Input: part model. Units: mm. Frame: model coordinates. A direction names the side the tool comes from. Coordinates: 2 decimals unless noted, no trailing zeros. Write each loop counter-clockwise with the first axis right and the second up, starting at its lowest first coordinate (ties: lowest second). Pieces come first, ordered by that corner, then holes. Notation, with made-up numbers: (63, 56) - (93, 56) arc R13 ccw to (93, 80) - close; hole circle Ø9 at (16.5, 73). An arc over 180 degrees is marked (long way). Put each result on its own line as item: value. Start each with the question number.
1. Pin query (flat end, axial travel): pin 1 (2 mm diameter, centred on x = -62, z = -5.5, fed in from +Y); pin 2 (1.5 mm diameter, centred on x = -2, z = -2.5, fed in from +Y); pin 3 (3 mm diameter, centred on x = -38.5, z = 1.5, fed in from +Y). Return the tip coordinate at first contact, or that it passes through.
2. Cut plane D-D, the plane x = -17. Return loops of the section in (y, z).
3. Cut plane A-A, the plane x = -64.35. Return loops of the section in (y, z).
4. Line query: line 1 (Y direction, x = -64.35, z = -20.8); line 2 (Y direction, x = -26, z = -21); line 3 (Z direction, x = -65, y = 8). Output: solid intervals per line, ascending.
5. Access query for faces 4 (the flat face through (-36, 7, 0)), 5 (the flat face through (-44.668, 13.675, -22.535)), 6 (the flat face through (-67, 48, -21)). Directions: +Z, -Z, +X, -X, +Y, -Y. A direction counts if a zero-diameter tool reaches every point of the face in a straight line with its end or side. Return the directions, or none.
6. Cut plane B-B, the plane y = 52.5. Return loops of the section in (x, z), and give its area (3 significant figures).
7. Pull-direction query (Z, two-part tool) for faces 1 (the flat face through (-68.48, 25.97, -22.54)), 2 (the flat face through (-3, 10, -15)), 3 (the flat face through (-3, 13, 2)); classes: released by +Z, released by -Z, zero draft, split by the parting line, or undercut.
8. Cut plane C-C, the plane z = -1.5. Return loops of the section in (x, y).
from build123d import *

# Parameters (mm, degrees)
SKETCH2_W            = 70
SKETCH2_H            = 20
BOSS_EXTRUDE1_DEPTH  = 5
SKETCH3_W            = 70
SKETCH3_H            = 5
BOSS_EXTRUDE2_DEPTH  = 10
SKETCH4_W            = 5
SKETCH4_H            = 5
BOSS_EXTRUDE3_DEPTH  = 10
LOFT1_START          = -5
LOFT1_DEPTH          = 5
SKETCH7_W            = 3
SKETCH7_H            = 20
BOSS_EXTRUDE4_DEPTH  = 5
LOFT2_START          = -5
LOFT2_DEPTH          = 5
BOSS_EXTRUDE5_DEPTH  = 5
SKETCH12_W           = 46.347010245
SKETCH12_H           = 26.5
CUT_EXTRUDE1_DEPTH   = 14
BOSS_EXTRUDE6_DEPTH  = 5
BOSS_EXTRUDE7_DEPTH  = 5
SKETCH17_W           = 6.7
SKETCH17_H           = 6
BOSS_EXTRUDE8_DEPTH  = 5
SKETCH18_W           = 5.3
SKETCH18_H           = 6
BOSS_EXTRUDE9_DEPTH  = 5
SKETCH23_W           = 6.7
SKETCH23_H           = 2
SKETCH23_W_2         = 5.3
BOSS_EXTRUDE12_DEPTH = 10
SKETCH24_R           = 1.6
CUT_EXTRUDE4_DEPTH   = 10


# Read off the part's stored shape, not the designer's step: Loft1, Loft2
with BuildPart() as part:
    # Sketch2 → Boss-Extrude1 (new body)
    with BuildSketch(Plane(origin=(0, 0, 0), x_dir=(1, 0, 0), z_dir=(0, 1, 0))):
        with Locations((-35, 10)):
            Rectangle(SKETCH2_W, SKETCH2_H)
    extrude(amount=BOSS_EXTRUDE1_DEPTH)

    # Sketch3 → Boss-Extrude2 (add)
    with BuildSketch(Plane(origin=(0, 0, 0), x_dir=(1, 0, 0), z_dir=(0, 1, 0))):
        with Locations((-35, 22.5)):
            Rectangle(SKETCH3_W, SKETCH3_H)
        with Locations((-35, -2.5)):
            Rectangle(SKETCH3_W, SKETCH3_H)
    extrude(amount=BOSS_EXTRUDE2_DEPTH)

    # Sketch4 → Boss-Extrude3 (add)
    with BuildSketch(Plane(origin=(0, 5, 0), x_dir=(1, 0, 0), z_dir=(0, 1, 0))):
        with Locations((-2.5, 2.5)):
            Rectangle(SKETCH4_W, SKETCH4_H)
        with Locations((-2.5, 17.5)):
            Rectangle(SKETCH4_W, SKETCH4_H)
    extrude(amount=BOSS_EXTRUDE3_DEPTH)

    # Loft1 outline → Loft1 (add)
    with BuildSketch(Plane.YZ.offset(LOFT1_START)):
        Polygon((15, 0), (10, 5), (10, 0), align=None)
    extrude(amount=LOFT1_DEPTH)

    # Sketch7 → Boss-Extrude4 (add)
    with BuildSketch(Plane(origin=(0, 5, 0), x_dir=(1, 0, 0), z_dir=(0, 1, 0))):
        with Locations((-68.5, 10)):
            Rectangle(SKETCH7_W, SKETCH7_H)
    extrude(amount=BOSS_EXTRUDE4_DEPTH)

    # Loft2 outline → Loft2 (add)
    with BuildSketch(Plane.YZ.offset(LOFT2_START)):
        Polygon((10, -25), (15, -20), (10, -20), align=None)
    extrude(amount=LOFT2_DEPTH)

    # Sketch10 → Boss-Extrude5 (add)
    with BuildSketch(Plane(origin=(0, 0, -25), x_dir=(-1, 0, 0), z_dir=(0, 0, -1))):
        Polygon((0, 10), (0, 41.5), (67, 41.5), (70, 10), align=None)
    extrude(amount=-BOSS_EXTRUDE5_DEPTH)

    # Sketch12 → Cut-Extrude1 (cut)
    with BuildSketch(Plane(origin=(0, 0, -25), x_dir=(-1, 0, 0), z_dir=(0, 0, -1))):
        with Locations((33.173505123, 23.25)):
            Rectangle(SKETCH12_W, SKETCH12_H)
    extrude(amount=-CUT_EXTRUDE1_DEPTH, mode=Mode.SUBTRACT)

    # Sketch13 → Boss-Extrude6 (add)
    with BuildSketch(Plane(origin=(0, 0, -25), x_dir=(-1, 0, 0), z_dir=(0, 0, -1))):
        Polygon((15, 30), (51.347010245, 10), (56.347010245, 10), (56.347010245, 13.748742075), (51.347010245, 16.5), (15, 36.5), (10, 36.5), (10, 32.751257925), align=None)
    extrude(amount=-BOSS_EXTRUDE6_DEPTH)

    # Sketch14 → Boss-Extrude7 (add)
    with BuildSketch(Plane(origin=(0, 0, -25), x_dir=(-1, 0, 0), z_dir=(0, 0, -1))):
        Polygon((35.673505122, 36.5), (33.173505122, 36.5), (33.173505122, 10), (38.173505122, 10), (38.173505122, 36.5), align=None)
    extrude(amount=-BOSS_EXTRUDE7_DEPTH)

    # Sketch17 → Boss-Extrude8 (add)
    with BuildSketch(Plane(origin=(0, 0, -25), x_dir=(-1, 0, 0), z_dir=(0, 0, -1))):
        with Locations((3.35, 44.5)):
            Rectangle(SKETCH17_W, SKETCH17_H)
    extrude(amount=-BOSS_EXTRUDE8_DEPTH)

    # Sketch18 → Boss-Extrude9 (add)
    with BuildSketch(Plane(origin=(0, 0, -25), x_dir=(-1, 0, 0), z_dir=(0, 0, -1))):
        with Locations((64.35, 44.5)):
            Rectangle(SKETCH18_W, SKETCH18_H)
    extrude(amount=-BOSS_EXTRUDE9_DEPTH)

    # Sketch23 → Boss-Extrude12 (add)
    with BuildSketch(Plane(origin=(0, 47.5, 0), x_dir=(1, 0, 0), z_dir=(0, 1, 0))):
        with Locations((-3.35, 21)):
            Rectangle(SKETCH23_W, SKETCH23_H)
        with Locations((-64.35, 21)):
            Rectangle(SKETCH23_W_2, SKETCH23_H)
    extrude(amount=BOSS_EXTRUDE12_DEPTH)

    # Sketch24 → Cut-Extrude4 (cut)
    with BuildSketch(Plane(origin=(0, 0, -22), x_dir=(-1, 0, 0), z_dir=(0, 0, -1))):
        with Locations((3.35, 52.5)):
            Circle(SKETCH24_R)
        with Locations((64.35, 52.5)):
            Circle(SKETCH24_R)
    extrude(amount=-CUT_EXTRUDE4_DEPTH, mode=Mode.SUBTRACT)


solid = part.part
Report:
1. pin 1: stops at y = 5
1. pin 2: stops at y = 15
1. pin 3: stops at y = 10
2. outline: (0, -25) - (10, -25) - (10, -20) - (5, -20) - (5, 0) - (10, 0) - (10, 5) - (0, 5) - close; (28.9, -25) - (35.4, -25) - (35.4, -20) - (28.9, -20) - close; (36.5, -25) - (41.5, -25) - (41.5, -20) - (36.5, -20) - close
3. outline: (0, -25) - (47.5, -25) - (47.5, -22) - (50.9, -22) - (50.9, -20) - (5, -20) - (5, 0) - (10, 0) - (10, 5) - (0, 5) - close; (54.1, -22) - (57.5, -22) - (57.5, -20) - (54.1, -20) - close
4. line 1: y = 0 to 50.9, 54.1 to 57.5
4. line 2: y = 0 to 10, 23.95 to 30.45, 36.5 to 41.5
4. line 3: z = -25 to -20, 0 to 5
5. face 4: +Y
5. face 5: +Z, -Z
5. face 6: +Z, -Z, -X, +Y
6. outline: (-67, -22) - (-65.95, -22) - (-65.95, -20) - (-67, -20) - close; (-62.75, -22) - (-61.7, -22) - (-61.7, -20) - (-62.75, -20) - close; (-6.7, -22) - (-4.95, -22) - (-4.95, -20) - (-6.7, -20) - close; (-1.75, -22) - (0, -22) - (0, -20) - (-1.75, -20) - close
6. area: 11.2 mm^2
7. face 1: zero draft
7. face 2: undercut
7. face 3: released by +Z
8. outline: (-70, 0) - (0, 0) - (0, 15) - (-5, 15) - (-5, 5) - (-67, 5) - (-67, 10) - (-70, 10) - close
